Design review of the part built by this model. Coordinates are the model's own, in mm. Round coordinates to 2 decimals unless told otherwise and drop trailing zeros. Write each loop counter-clockwise with the first axis right and the second up, starting at its lowest first coordinate (ties: lowest second). Pieces come first, ordered by that corner, then holes.
Autodesk Inventor part; units mm, degrees
ref_plane "YZ Plane" through (0, 0, 0) normal (1, 0, 0) x (0, 1, 0)
ref_plane "XZ Plane" through (0, 0, 0) normal (0, 1, 0) x (-1, 0, 0)
ref_plane "XY Plane" through (0, 0, 0) normal (0, 0, 1) x (1, 0, 0)
sketch "スケッチ1" plane through (0, 0, 0) normal (0, 0, 1) x (1, 0, 0)
  line L0 (7.5, 7.5) -> (-7.5, 7.5)
  line L1 (-7.5, 7.5) -> (-7.5, -7.5)
  line L2 (-7.5, -7.5) -> (7.5, -7.5)
  line L3 (7.5, -7.5) -> (7.5, 7.5)
  line L4 (7.5, 7.5) -> (-7.5, -7.5) construction
  line L5 (-7.5, 7.5) -> (7.5, -7.5) construction
  line L6 (-6, 6) -> (6, 6)
  line L7 (6, 6) -> (6, -6)
  line L8 (6, -6) -> (-6, -6)
  line L9 (-6, -6) -> (-6, 6)
  point P0 (0, 0)
  dimension "d0" = 15
  dimension "d1" = 15
  dimension "d2" = 1.5
extrude "押し出し1" add sketch "スケッチ1" along normal blind 1117
sketch "スケッチ2" plane through (-7.5, 7.5, 1117) normal (0, 1, 0) x (1, 0, 0)
  circle A0 centre (7.5, 1107) radius 1.6
  circle A1 centre (7.5, 1097) radius 1.6
  line L0 (15, 1117) -> (0, 1117)
  circle A2 centre (7.5, 10) radius 1.6
  circle A3 centre (7.5, 20) radius 1.6
  line L1 (15, 0) -> (0, 0)
  point P0 (7.5, 1117)
  point P1 (7.5, 1117)
  point P2 (7.5, 0)
  dimension "d5" = 3.2
  dimension "d6" = 3.2
  dimension "d7" = 10
  dimension "d8" = 10
  dimension "d9" = 3.2
  dimension "d10" = 3.2
  dimension "d11" = 10
  dimension "d12" = 10
extrude "押し出し2" cut sketch "スケッチ2" against normal through all
properties part number "上昇機構_角柱2" material "アルミニウム 6061"
1) Add section B-B on y = 3.5. State the section outline as (x, z) points, and give its area (3 significant figures).
2) For line 1 along Z through (x, y) = (0, 6.55); line 2 along X through (y, z) = (4.25, 573.5), list the stretches that pass through material, from the lowest coordinate up.
3) Add section A-A on z = 225. State the section outline as (x, y) points, and give its area (3 significant figures).
4) For P1, Ø3, axis at x = 0, z = 10, coming from the +Y side; P2, Ø5, axis at x = 0, z = 1107, coming from the -Y side, all flat-tipped, find the tip position at first contact; note any pin that passes through.
Computed:
1. outline: (-7.5, 0) - (-6, 0) - (-6, 1117) - (-7.5, 1117) - close; (6, 0) - (7.5, 0) - (7.5, 1117) - (6, 1117) - close
1. area: 3,350 mm2
2. line 1: z = 0 to 8.4, 11.6 to 18.4, 21.6 to 1095.4, 1098.6 to 1105.4, 1108.6 to 1117
2. line 2: x = -7.5 to -6, 6 to 7.5
3. outline: (-7.5, -7.5) - (7.5, -7.5) - (7.5, 7.5) - (-7.5, 7.5) - close; hole (-6, -6) - (6, -6) - (6, 6) - (-6, 6) - close
3. area: 81.0 mm2
4. P1: passes through
4. P2: stops at y = -7.5
